```python
from build123d import *

# Parameters (mm, degrees)
SKETCH1_R           = 50
BOSS_EXTRUDE1_DEPTH = 105
BOSS_EXTRUDE3_START = -10
SKETCH2_R           = 50
SKETCH2_W           = 100
SKETCH2_H           = 150
BOSS_EXTRUDE3_DEPTH = 10
SKETCH3_R           = 5
CUT_EXTRUDE1_DEPTH  = 10
FILLET1_R           = 50


with BuildPart() as part:
    # Sketch1 → Boss-Extrude1 (new, symmetric)
    with BuildSketch(Plane.XY):
        Circle(SKETCH1_R)
    extrude(amount=BOSS_EXTRUDE1_DEPTH, both=True)

    # Sketch2 → Boss-Extrude3 (add)
    with BuildSketch(Plane(origin=(0, 0, -105), x_dir=(-1, 0, 0), z_dir=(0, 0, -1)).offset(BOSS_EXTRUDE3_START)):
        Circle(SKETCH2_R)
        with BuildLine():
            Line((0, 75), (0, -75))
            ThreePointArc((0, -75), (75, 0), (0, 75))
        make_face()
        with Locations((-50, 0)):
            Rectangle(SKETCH2_W, SKETCH2_H)
    extrude(amount=BOSS_EXTRUDE3_DEPTH)

    # Sketch3 → Cut-Extrude1 (cut)
    with BuildSketch(Plane(origin=(0, 0, -105), x_dir=(-1, 0, 0), z_dir=(0, 0, -1))):
        with Locations((0, 62.5)):
            Circle(SKETCH3_R)
        with Locations((62.5, 0)):
            Circle(SKETCH3_R)
        with Locations((0, -62.5)):
            Circle(SKETCH3_R)
    extrude(amount=-CUT_EXTRUDE1_DEPTH, mode=Mode.SUBTRACT)

    # Fillet1
    fillet1_edges = [part.edges().sort_by_distance(p)[0] for p in [
        (100, -75, -100),
        (100, 75, -100),
    ]]
    fillet(fillet1_edges, radius=FILLET1_R)


solid = part.part
```
CAD build for the part. Positions are in the model's coordinates, mm. A direction names the side the tool comes from. Round coordinates to 2 decimals unless told otherwise and drop trailing zeros. Order: outer loops, then holes, each group sorted by start corner. A loop starts at its lowest first (then second) coordinate and runs counter-clockwise, first axis right, second up. Notation, with made-up numbers: (4, -5.75) - (43, -5.75) arc R29 ccw to (43, 31.25) - close; hole circle Ø6 at (-31, 33.5). An arc over 180 degrees is marked (long way). Use CSV: the item, a comma, the result in double quotes. Start each with the question number.
1) Saw through at A-A (y = 0). List the corners of the cut face in (x, z).
2) Wall check: L1, parallel to Y at x = 0, z = -97.25; L2, parallel to Z at x = -51, y = -46; L3, parallel to Y at x = -62, z = -98. Give the ranges that are in metal, low to high. Write a range as [from, to].
3) Saw through at D-D (x = 27.5). List the corners of the cut face in (y, z), and give its area (3 significant figures).
4) Saw through at C-C (z = 33). List the corners of the cut face in (x, y), and give its area (3 significant figures).
5) Saw through at B-B (x = -62.5). List the corners of the cut face in (y, z), and give its area (3 significant figures).
6) Tool access for faces 4 (the cylindrical face through (-74.98, -1.65, -99.93)), 5 (the cylindrical face through (47.69, 15.02, 6.4)): list every direction of +Z, -Z, +X, -X, +Y, -Y with a clear straight run to the whole face (end or side of a thin tool).
7) Two-plate mould, pull along Y, no slides. Class faces 1 (the flat face through (-1, 1, 105)), 2 (the cylindrical face through (-2.688, 66.716, -100.07)), 3 (the cylindrical face through (84.964, -60.742, -100.07)): pulls with the +Y half, pulls with the -Y half, needs draft (parallel to the pull), parting line crosses it, or undercut.
8) Pin check, flat tips, straight feed: pin 1 Ø1.5 at (y, z) = (-22, 44.5) entering from -X; pin 2 Ø3 at (x, z) = (10.5, -3) entering from +Y; pin 3 Ø4 at (x, y) = (48.5, -19.5) entering from +Z; pin 4 Ø8 at (x, y) = (0, 62.5) entering from +Z. Stop position of each tip, or through.
Values follow:
1,outline,"(-75, -105) - (-67.5, -105) - (-67.5, -95) - (-75, -95) - close; (-57.5, -105) - (100, -105) - (100, -95) - (50, -95) - (50, 105) - (-50, 105) - (-50, -95) - (-57.5, -95) - close"
2,L1,"y = [-75, -67.5], [-57.5, 57.5], [67.5, 75]"
2,L2,"z = [-105, -95]"
2,L3,"y = [-42.2, -4.97], [4.97, 42.2]"
3,outline,"(-75, -105) - (75, -105) - (75, -95) - (41.76, -95) - (41.76, 105) - (-41.76, 105) - (-41.76, -95) - (-75, -95) - close"
3,area,"18,200 mm2"
4,outline,"circle Ø100 at (0, 0)"
4,area,"7,850 mm2"
5,outline,"(-41.46, -105) - (-5, -105) - (-5, -95) - (-41.46, -95) - close; (5, -105) - (41.46, -105) - (41.46, -95) - (5, -95) - close"
5,area,"729 mm2"
6,face 4,"+Z, -Z, -X"
6,face 5,"+Z"
7,face 1,"needs draft"
7,face 2,"undercut"
7,face 3,"pulls with the -Y half"
8,pin 1,"stops at x = -45.26"
8,pin 2,"stops at y = 49.18"
8,pin 3,"stops at z = -95"
8,pin 4,"passes through"
